Geometry check sheet. Reference: the model listing, model coordinates, mm. Face numbers are marked on the shaded views. A direction names the side the tool comes from. Give positions to 0.01 mm unless a question says otherwise; leave off trailing zeros. Loops run counter-clockwise (first coordinate to the right, second up) from the corner with the lowest first, then second, coordinate; pieces in that order, holes last.
```python
from build123d import *

# Parameters (mm, degrees)
F1_DEPTH = 1
F3_DEPTH = 12
F5_DEPTH = 1


with BuildPart() as f1:
    # F0 (on Top) → F1 (new body)
    with BuildSketch(Plane.XY):
        Polygon((-115, -42.5), (115, -42.5), (115, 42.5), (-57, 42.5), (-115, -15.5), align=None)
    extrude(amount=F1_DEPTH)

    # F2 (on face) → F3 (join)
    with BuildSketch(Plane(origin=(0, 0, 0), x_dir=(1, 0, 0), z_dir=(0, 0, -1))):
        Polygon((-115, 42.5), (-115, 15.5), (-57, -42.5), (115, -42.5), (115, 42.5), (114, 42.5), (114, -41.5), (-56.5857864376, -41.5), (-114, 15.9142135624), (-114, 42.5), align=None)
    extrude(amount=F3_DEPTH)

    # F4 (on face) → F5 (cut)
    with BuildSketch(Plane(origin=(-49.75, 49.75, 0), x_dir=(-0.7071067812, -0.7071067812, 0), z_dir=(-0.7071067812, 0.7071067812, 0))):
        Polygon((10.2630483272, 1), (10.2530483272, 1), (10.2530483272, -12), (23.2630483272, -12), align=None)
        Polygon((92.2774349448, -12), (92.2774349448, 1), (92.2674349448, 1), (79.2674349448, -12), align=None)
    extrude(amount=-F5_DEPTH, mode=Mode.SUBTRACT)


solid = f1.part
```
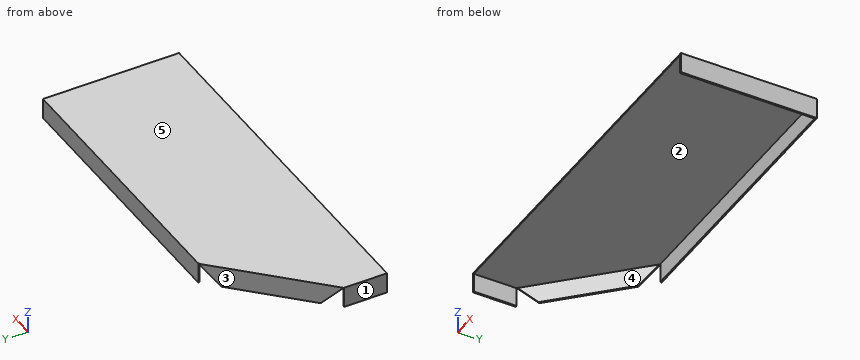
1) Mould release check, pull along X, two halves, no side actions. Record for the marked faces 3, 4 and 5: +X half, -X half, draft (parallel to the pull), parting line (faces both ways), or undercut.
2) Sectioned sample at B-B on z = -6.5. Enter the section's corners in (x, y).
3) Depth check by flat-ended pin: P1, Ø3, axis at x = -88.5, z = -10, coming from the +Y side; P2, Ø5, axis at x = 37, y = -24.5, coming from the -Z side; P3, Ø3, axis at x = 21, z = -2, coming from the -Y side. Enter the tip coordinate at first touch or a pass-through.
4) Tool access check on the marked faces 1 and 2. Record the directions out of +Z, -Z, +X, -X, +Y, -Y that give a thin tool (end or side, any length) a straight path to the whole face; none if there is none.
5) Sectioned sample at C-C on x = -86.5. Enter the section's corners in (y, z), plus the area to 3 significant figures.
6) Sectioned sample at A-A on y = -21. Enter the section's corners in (x, z).
7) Sectioned sample at D-D on y = 28.5. Enter the section's corners in (x, z).
8) Scan lines: line 1 along X through (y, z) = (-24.5, -5.25); line 2 along Z through (x, y) = (1.5, 34); line 3 along X through (y, z) = (20, -8.5). Record each from-to range of solid material in increasing order.
Determined:
1. face 3: -X half
1. face 4: undercut
1. face 5: draft
2. outline: (-115, -42.5) - (-114, -42.5) - (-114, -15.91) - (-114.29, -16.21) - (-115, -15.5) - close; (-109.69, -10.19) - (-108.98, -10.9) - (-61.6, 36.48) - (-62.31, 37.19) - close; (-57, 42.5) - (-56.29, 41.79) - (-56.59, 41.5) - (114, 41.5) - (114, -42.5) - (115, -42.5) - (115, 42.5) - close
3. P1: stops at y = 12.5
3. P2: stops at z = 0
3. P3: stops at y = 41.5
4. face 1: +Z, -Z, -X, +Y, -Y
4. face 2: -Z, -Y
5. outline: (-42.5, 0) - (11.59, 0) - (11.59, -12) - (13, -12) - (13, 1) - (-42.5, 1) - close
5. area: 72.5 mm2
6. outline: (-115, -12) - (-114, -12) - (-114, 0) - (114, 0) - (114, -12) - (115, -12) - (115, 1) - (-115, 1) - close
7. outline: (-71, -12) - (-69.59, -12) - (-69.59, 0) - (114, 0) - (114, -12) - (115, -12) - (115, 1) - (-71, 1) - close
8. line 1: x = -115 to -114, 114 to 115
8. line 2: z = 0 to 1
8. line 3: x = -79.5 to -78.09, 114 to 115
